Here's how the part is built. I have some questions about the finished solid (model axes, mm). A direction names the side the tool comes from. Give positions to 0.01 mm unless a question says otherwise; leave off trailing zeros. Write each loop counter-clockwise with the first axis right and the second up, starting at its lowest first coordinate (ties: lowest second). Pieces come first, ordered by that corner, then holes. Notation, with made-up numbers: (-34.5, 85.25) -> (-0.5, 85.25) arc R21 cw to (-0.5, 116.25) -> close; hole circle Ø1 at (51, 18). An arc over 180 degrees is marked (long way). Return JSON: item names as keys, results as strings.
from build123d import *

# Parameters (mm, degrees)
F0_W      = 63.5
F0_H      = 38.1
F1_DEPTH  = 6.35
F2_R      = 3.175
F3_DEPTH  = 25.4
F4_W      = 25.4
F4_H      = 12.7
F5_DEPTH  = 31.75
F6_R      = 6.35
F7_DEPTH  = 25.4
F8_R      = 9.525
F9_W      = 12.7
F9_H      = 12.7
F10_DEPTH = 12.7
F12_DEPTH = 25.4


with BuildPart() as f1:
    # F0 (on Top) → F1 (new body)
    with BuildSketch(Plane.XY):
        with Locations((-38.658564874, 19.05)):
            Rectangle(F0_W, F0_H)
    extrude(amount=F1_DEPTH)

    # F2 (on face) → F3 (cut)
    with BuildSketch(Plane.XY.offset(6.35)):
        with Locations((-16.433564874, 28.575)):
            Circle(F2_R)
        with Locations((-16.433564874, 9.525)):
            Circle(F2_R)
        with Locations((-60.883564874, 9.525)):
            Circle(F2_R)
    extrude(amount=-F3_DEPTH, mode=Mode.SUBTRACT)

    # F4 (on face) → F5 (join)
    with BuildSketch(Plane.XY.offset(6.35)):
        with Locations((-57.708564874, 31.75)):
            Rectangle(F4_W, F4_H)
    extrude(amount=F5_DEPTH)

    # F6 (on face) → F7 (cut)
    with BuildSketch(Plane.XZ.offset(-25.4)):
        with Locations((-57.708564874, 25.4)):
            Circle(F6_R)
        with BuildLine():
            ThreePointArc((-70.408564874, 25.4), (-57.708564874, 37.7975720317), (-45.008564874, 25.4))
            Line((-45.008564874, 25.4), (-45.008564874, 38.1))
            Line((-45.008564874, 38.1), (-70.408564874, 38.1))
            Line((-70.408564874, 38.1), (-70.408564874, 25.4))
        make_face()
    extrude(amount=-F7_DEPTH, mode=Mode.SUBTRACT)

    # F8
    f8_edges = [f1.edges().sort_by_distance(p)[0] for p in [
        (-6.908565, 0, 3.175),
        (-70.408565, 0, 3.175),
    ]]
    fillet(f8_edges, radius=F8_R)

    # F9 (on face) → F10 (join)
    with BuildSketch(Plane.YZ.offset(-45.008564874)):
        with Locations((31.75, 12.7)):
            Rectangle(F9_W, F9_H)
    extrude(amount=F10_DEPTH)

    # F11 (on face) → F12 (cut)
    with BuildSketch(Plane.XZ.offset(-25.4)):
        with BuildLine():
            Line((-32.308564874, 19.05), (-38.658564874, 19.05))
            ThreePointArc((-38.658564874, 19.05), (-34.1684368135, 17.1901280605), (-32.308564874, 12.7))
            Line((-32.308564874, 12.7), (-32.308564874, 19.05))
        make_face()
        with BuildLine():
            Line((-38.658564874, 19.05), (-45.008564874, 19.05))
            Line((-45.008564874, 19.05), (-45.008564874, 12.7))
            ThreePointArc((-45.008564874, 12.7), (-43.1486929345, 17.1901280605), (-38.658564874, 19.05))
        make_face()
        with BuildLine():
            ThreePointArc((-32.308564874, 12.7), (-34.1684368135, 8.2098719395), (-38.658564874, 6.35))
            Line((-38.658564874, 6.35), (-32.308564874, 6.35))
            Line((-32.308564874, 6.35), (-32.308564874, 12.7))
        make_face()
        with BuildLine():
            ThreePointArc((-38.658564874, 19.05), (-43.1486929345, 17.1901280605), (-45.008564874, 12.7))
            ThreePointArc((-45.008564874, 12.7), (-43.1486929345, 8.2098719395), (-38.658564874, 6.35))
            ThreePointArc((-38.658564874, 6.35), (-34.1684368135, 8.2098719395), (-32.308564874, 12.7))
            ThreePointArc((-32.308564874, 12.7), (-34.1684368135, 17.1901280605), (-38.658564874, 19.05))
        make_face()
    extrude(amount=-F12_DEPTH, mode=Mode.SUBTRACT)


solid = f1.part
1. Suppose I cut it at D-D, the plane y = 15.5. List the corners of the cut face in (x, z) for me, and give its area (3 significant figures).
Taken from the geometry:
{"outline": "(-70.41, 0) -> (-6.91, 0) -> (-6.91, 6.35) -> (-70.41, 6.35) -> close", "area": "403 mm²"}
2. Suppose I cut it at B-B, the plane z = 22.5. List the corners of the cut face in (x, y) for me.
Taken from the geometry:
{"outline": "(-70.41, 25.4) -> (-63.36, 25.4) -> (-63.36, 38.1) -> (-70.41, 38.1) -> close; (-52.06, 25.4) -> (-45.01, 25.4) -> (-45.01, 38.1) -> (-52.06, 38.1) -> close"}
3. For pin 1 Ø3 at (x, y) = (-63, 12) entering from +Z; pin 2 Ø14.5 at (x, z) = (-57.71, 25.4) entering from -Y; pin 3 Ø4 at (x, z) = (-26, 7.5) entering from +Y; pin 4 Ø14 at (y, z) = (29, 21) entering from +X, each with a flat end and sliding along its axis, tell me the tip position at first contact or that it passes through.
Taken from the geometry:
{"pin 1": "stops at z = 6.35", "pin 2": "stops at y = 25.4", "pin 3": "stops at y = 38.1", "pin 4": "stops at x = -45.01"}
4. Suppose I cut it at C-C, the plane x = -46.5. List the corners of the cut face in (y, z) for me.
Taken from the geometry:
{"outline": "(0, 0) -> (38.1, 0) -> (38.1, 31.07) -> (25.4, 31.07) -> (25.4, 6.35) -> (0, 6.35) -> close"}
5. If I drill on line 1 (X direction, y = 7.5, z = 6); line 2 (X direction, y = 28.5, z = 25); line 3 (Z direction, x = -12, y = 5), over which ranges is the centre line in solid material (lowest first)? Write a range as [from, to].
Taken from the geometry:
{"line 1": "x = [-70.19, -63.33], [-58.44, -18.88], [-13.99, -7.13]", "line 2": "x = [-70.41, -64.05], [-51.37, -45.01]", "line 3": "z = [0, 6.35]"}
6. If we mould it in two halves opening along Y, with no side actions, what happens to faces 4 (the face through (-67.69, 2.86, 3.22)), 5 (the face through (-70.409, 30, 10)), 6 (the face through (-57.855, 10.479, 3.219))? For each: released by +Y, released by -Y, zero draft, split by the parting line, or undercut.
Taken from the geometry:
{"face 4": "released by -Y", "face 5": "zero draft", "face 6": "undercut"}
7. Which directions (+Z, -Z, +X, -X, +Y, -Y) give clear straight access to the entire face, cutting with the end or side of a thin tool? Please do faces 1 (the face through (-45.009, 32, 19)), 2 (the face through (-32, 15, 6.35)), 3 (the face through (-58, 25.4, 18)).
Taken from the geometry:
{"face 1": "+Z, +X, +Y, -Y", "face 2": "+Z, +X, -Y", "face 3": "+Z, +X, -X, -Y"}
